from build123d import *

# Parameters (mm, degrees)
BOSS_EXTRUDE1_DEPTH = 3
SKETCH2_R           = 3.5
CUT_EXTRUDE1_DEPTH  = 159.793104384
CUT_EXTRUDE3_DEPTH  = 159.793104384
BOSS_EXTRUDE2_START = -3
SKETCH10_R          = 3.5
BOSS_EXTRUDE2_DEPTH = 3
SKETCH11_R          = 1.5
CUT_EXTRUDE4_DEPTH  = 10


with BuildPart() as part:
    # Sketch1 → Boss-Extrude1 (new body)
    with BuildSketch(Plane(origin=(0, 0, 0), x_dir=(1, 0, 0), z_dir=(0, 1, 0))):
        with BuildLine():
            Line((140.3125, 17.497209599), (0.357142857, 19.99681097))
            ThreePointArc((0.357142857, 19.99681097), (-19.999202727, 0.178578547), (0, -20))
            Line((0, -20), (140, -17.5))
            ThreePointArc((140, -17.5), (157.499302386, -0.156256229), (140.3125, 17.497209599))
        make_face()
    extrude(amount=BOSS_EXTRUDE1_DEPTH)

    # Sketch2 → Cut-Extrude1 (cut, through all)
    with BuildSketch(Plane(origin=(0, 3, 0), x_dir=(1, 0, 0), z_dir=(0, 1, 0))):
        with Locations(Location((0, 0, 0), (0, 0, 270))):
            Circle(SKETCH2_R)
        with Locations(Location((140, 0, 0), (0, 0, 270))):
            Circle(SKETCH2_R)
    extrude(amount=-CUT_EXTRUDE1_DEPTH, mode=Mode.SUBTRACT)

    # Sketch4 → Cut-Extrude3 (cut, through all)
    with BuildSketch(Plane(origin=(0, 3, 0), x_dir=(1, 0, 0), z_dir=(0, 1, 0))):
        with BuildLine():
            ThreePointArc((101.494647455, -6.185682468), (107.64017994, 0.394224207), (101.283865867, 6.770744637))
            Line((101.283865867, 6.770744637), (29.173044697, 8.058643229))
            ThreePointArc((29.173044697, 8.058643229), (21.397292905, 0.29833633), (29.157599804, -7.477415462))
            Line((29.157599804, -7.477415462), (101.052392136, -6.193579885))
            Line((101.052392136, -6.193579885), (101.494647455, -6.185682468))
        make_face()
    extrude(amount=-CUT_EXTRUDE3_DEPTH, mode=Mode.SUBTRACT)

    # Sketch10 → Boss-Extrude2 (add)
    with BuildSketch(Plane(origin=(0, 3, 0), x_dir=(1, 0, 0), z_dir=(0, 1, 0)).offset(BOSS_EXTRUDE2_START)):
        with BuildLine():
            Line((-0.353982548, 19.996867164), (-39.998419596, 19.999999875))
            Line((-39.998419596, 19.999999875), (-40, 20))
            ThreePointArc((-40, 19.999999938), (-59.999999938, -3.1e-08), (-40, -20))
            Line((-40, -20), (0, -20))
            ThreePointArc((0, -20), (-19.999216776, -0.176998206), (-0.353982548, 19.996867164))
        make_face()
        with Locations(Location((-40, 0, 0), (0, 0, 270))):
            Circle(SKETCH10_R, mode=Mode.SUBTRACT)
    extrude(amount=BOSS_EXTRUDE2_DEPTH)

    # Sketch11 → Cut-Extrude4 (cut)
    with BuildSketch(Plane(origin=(0, 3, 0), x_dir=(1, 0, 0), z_dir=(0, 1, 0))):
        with Locations(Location((40.994069635, 12.848317219, 0), (0, 0, 270))):
            Circle(SKETCH11_R)
        with Locations(Location((40.994069635, -12.26684706, 0), (0, 0, 270))):
            Circle(SKETCH11_R)
        with Locations(Location((100.994069635, -12.26684706, 0), (0, 0, 270))):
            Circle(SKETCH11_R)
        with Locations(Location((100.994069635, 12.848317219, 0), (0, 0, 270))):
            Circle(SKETCH11_R)
    extrude(amount=-CUT_EXTRUDE4_DEPTH, mode=Mode.SUBTRACT)


solid = part.part
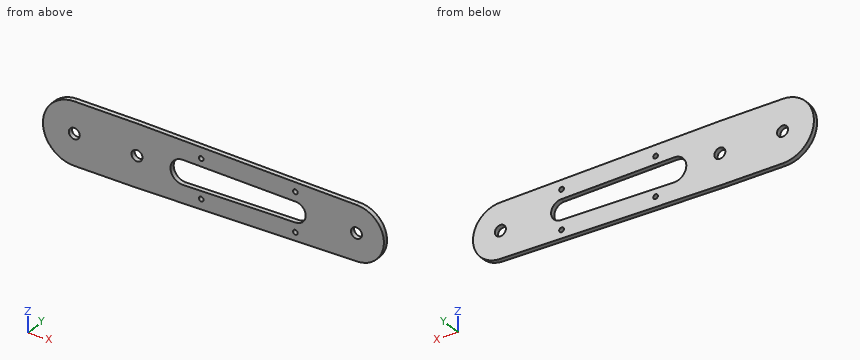
The model under review builds one solid part; all positions refer to its coordinate system, in mm. Coordinates: 2 decimals unless noted, no trailing zeros. Loops run counter-clockwise (first coordinate to the right, second up) from the corner with the lowest first, then second, coordinate; pieces in that order, holes last. Notation, with made-up numbers: M -1.5,-26 L 33.5,-26 A27 ccw 33.5,1 Z; hole C -35,-13.5 d9. An arc over 180 degrees is marked long. Put each result on its own line as item: value. Start each with the question number.
Q1. Add section A-A (z = 0). Write out the cut boundary in (x, y), and give its area (3 significant figures).
Q2. Clearance check with flat-ended pins moving along their axes: pin 1 (1 mm diameter, centred on x = 81, y = 1, fed in from -Z); pin 2 (1 mm diameter, centred on y = 2, z = -1.5, fed in from +X); pin 3 (1 mm diameter, centred on x = 3.5, y = 2.5, fed in from +Z). State where each tip first meets the part, or that it passes through.
Q3. Wall thickness on line 1 (X direction, y = 1.95, z = 0); line 2 (X direction, y = 0.5, z = 13); line 3 (X direction, y = 1.15, z = 3): over which ranges is each line inside the solid? List them lowest first.
Q4. Add section C-C (y = 1.6). Count the separate pieces of the cut face and the enclosed holes in it, and give its area (3 significant figures).
Q5. Add section D-D (x = 119). Write out the cut boundary in (y, z) (3 decimals), and give its area (3 significant figures).
Q6. Add section B-B (x = 47). Write out the cut boundary in (y, z), and give its area (3 significant figures).
Answers:
1. outline: M -60,0 L -43.5,0 L -43.5,3 L -60,3 Z; M -36.5,0 L -3.5,0 L -3.5,3 L -36.5,3 Z; M 3.5,0 L 21.4,0 L 21.4,3 L 3.5,3 Z; M 107.63,0 L 136.5,0 L 136.5,3 L 107.63,3 Z; M 143.5,0 L 157.5,0 L 157.5,3 L 143.5,3 Z
1. area: 331 mm^2
2. pin 1: stops at z = -18.57
2. pin 2: stops at x = 157.47
2. pin 3: stops at z = 19.95
3. line 1: x = -60 to -43.5, -36.5 to -3.5, 3.5 to 21.4, 107.63 to 136.5, 143.5 to 157.5
3. line 2: x = -55.2 to 39.69, 42.3 to 99.69, 102.3 to 151.72
3. line 3: x = -59.77 to -41.8, -38.2 to -1.8, 1.8 to 22.13, 106.74 to 138.2, 141.8 to 157.24
4. separate pieces: 1
4. enclosed holes: 8
4. area: 6,630 mm^2
5. outline: M 0,-17.878 L 3,-17.878 L 3,17.875 L 0,17.875 Z
5. area: 107 mm^2
6. outline: M 0,-19.16 L 3,-19.16 L 3,-7.74 L 0,-7.74 Z; M 0,7.16 L 3,7.16 L 3,19.16 L 0,19.16 Z
6. area: 70.3 mm^2
